Read the model definition and answer for the solid it produces. Units are mm, in the model's axes. A direction names the side the tool comes from. Round coordinates to 2 decimals unless told otherwise and drop trailing zeros. Write each loop counter-clockwise with the first axis right and the second up, starting at its lowest first coordinate (ties: lowest second). Pieces come first, ordered by that corner, then holes.
from build123d import *

# Parameters (mm, degrees)
SKETCH1_W           = 25.4
SKETCH1_H           = 25.4
SKETCH1_W_2         = 21.4
SKETCH1_H_2         = 21.4
BOSS_EXTRUDE1_DEPTH = 110
SKETCH2_R           = 2
CUT_EXTRUDE1_DEPTH  = 26.4


with BuildPart() as part:
    # Sketch1 → Boss-Extrude1 (new body)
    with BuildSketch(Plane.XY):
        with Locations((12.7, 12.7)):
            Rectangle(SKETCH1_W, SKETCH1_H)
        with Locations((12.7, 12.7)):
            Rectangle(SKETCH1_W_2, SKETCH1_H_2, mode=Mode.SUBTRACT)
    extrude(amount=BOSS_EXTRUDE1_DEPTH)

    # Sketch2 → Cut-Extrude1 (cut, through all)
    with BuildSketch(Plane.XZ):
        with Locations((12.7, 98)):
            Circle(SKETCH2_R)
    extrude(amount=-CUT_EXTRUDE1_DEPTH, mode=Mode.SUBTRACT)


solid = part.part
Q1. Section D-D (x = 12.7) is taken. Determine the outline of the cut face in (y, z).
Verdict:
outline: (0, 0) - (2, 0) - (2, 96) - (0, 96) - close; (0, 100) - (2, 100) - (2, 110) - (0, 110) - close; (23.4, 0) - (25.4, 0) - (25.4, 96) - (23.4, 96) - close; (23.4, 100) - (25.4, 100) - (25.4, 110) - (23.4, 110) - close
Q2. Straight lines are drawn through the part: probe 1 along Y at (x, z) = (12.25, 14); probe 2 along Z at (x, y) = (12.7, 23.85). For each, find the intervals that lie inside material, in ascending order.
Verdict:
probe 1: y = 0 to 2, 23.4 to 25.4
probe 2: z = 0 to 96, 100 to 110
Q3. Which of the six approach directions +Z, -Z, +X, -X, +Y, -Y give full straight-line access (tool end or side, diameter ignored) to faces 4 (the cylindrical face through (12.44, 24.386, 99.983)), 5 (the flat face through (13, 23.4, 54))?
Verdict:
face 4: +Y, -Y
face 5: +Z, -Z
Q4. Section C-C (z = 98) is taken. Determine the outline of the cut face in (x, y).
Verdict:
outline: (0, 0) - (10.7, 0) - (10.7, 2) - (2, 2) - (2, 23.4) - (10.7, 23.4) - (10.7, 25.4) - (0, 25.4) - close; (14.7, 0) - (25.4, 0) - (25.4, 25.4) - (14.7, 25.4) - (14.7, 23.4) - (23.4, 23.4) - (23.4, 2) - (14.7, 2) - close
Q5. Determine the mould class of faces 1 (the flat face through (24, 13, 110)), 2 (the flat face through (0, 13, 54)), 3 (the cylindrical face through (12.44, 0.986, 99.983)) for opening direction X: pulls with the +X half, pulls with the -X half, needs draft (parallel to the pull), parting line crosses it, or undercut.
Verdict:
face 1: needs draft
face 2: pulls with the -X half
face 3: undercut
Q6. Section A-A (x = 7.5) is taken. Determine the outline of the cut face in (y, z), then the cut area to 3 significant figures.
Verdict:
outline: (0, 0) - (2, 0) - (2, 110) - (0, 110) - close; (23.4, 0) - (25.4, 0) - (25.4, 110) - (23.4, 110) - close
area: 440 mm2
